Design review of the part shown in the three views and the two pictorial views. Dimensions are in mm from the part's minimum x, y and z. Give positions to 0.01 mm unless a question says otherwise; leave off trailing zeros. Loops run counter-clockwise (first coordinate to the right, second up) from the corner with the lowest first, then second, coordinate; pieces in that order, holes last. Notation, with made-up numbers: M 0,-10 L 17,-10 A22 cw 17,16 Z; hole C 46,47 d3. An arc over 180 degrees is marked long. Return JSON: item names as keys, results as strings. Group by question number.
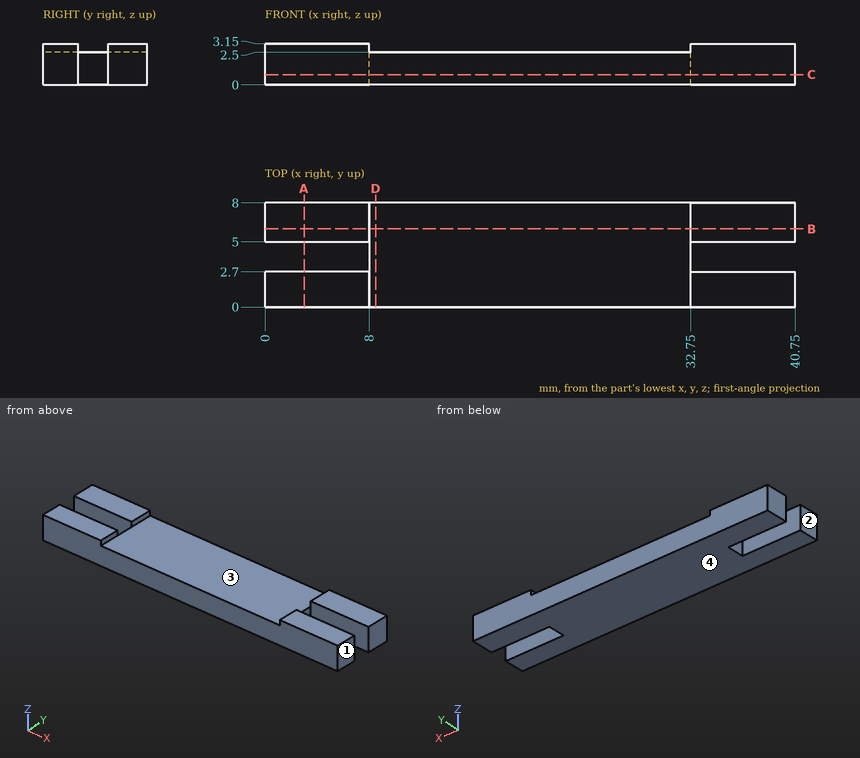
(1) For pin 1 (3 mm diameter, centred on x = 15.5, y = 6, fed in from +Z); pin 2 (1.8 mm diameter, centred on y = 3.5, z = 2, fed in from -X), all flat-tipped, find the tip position at first contact; note any pin that passes through.
(2) Add section C-C (z = 0.8). Write out the cut boundary in (x, y), and give its area (3 significant figures).
(3) For probe 1 along Y at (x, z) = (5, 0.85); probe 2 along X at (y, z) = (2.25, 2.95); probe 3 along Z at (x, y) = (19.5, 4.25), list the stretches that pass through material, from the lowest coordinate up.
(4) Add section D-D (x = 8.5). Write out the cut boundary in (y, z), and give its area (3 significant figures).
(5) Add section B-B (y = 6). Write out the cut boundary in (x, z), and give its area (3 significant figures).
(6) Mouldability with a two-part tool opening along X and no side actions: class the marked faces 1, 2, 3 and 4 as released by +X, released by -X, zero draft, split by the parting line, or undercut.
(7) Add section A-A (x = 3). Write out the cut boundary in (y, z).
Verdict:
{
 "1": {"pin 1": "stops at z = 2.5", "pin 2": "stops at x = 0"},
 "2": {"outline": "M 0,0 L 40.75,0 L 40.75,2.7 L 32.75,2.7 L 32.75,5 L 40.75,5 L 40.75,8 L 0,8 L 0,5 L 8,5 L 8,2.7 L 0,2.7 Z", "area": "289 mm²"},
 "3": {"probe 1": "y = 0 to 2.7, 5 to 8", "probe 2": "x = 0 to 8, 32.75 to 40.75", "probe 3": "z = 0 to 2.5"},
 "4": {"outline": "M 0,0 L 8,0 L 8,2.5 L 0,2.5 Z", "area": "20.0 mm²"},
 "5": {"outline": "M 0,0 L 40.75,0 L 40.75,3.15 L 32.75,3.15 L 32.75,2.5 L 8,2.5 L 8,3.15 L 0,3.15 Z", "area": "112 mm²"},
 "6": {"face 1": "released by +X", "face 2": "released by -X", "face 3": "undercut", "face 4": "zero draft"},
 "7": {"outline": "M 0,0 L 2.7,0 L 2.7,3.15 L 0,3.15 Z; M 5,0 L 8,0 L 8,3.15 L 5,3.15 Z"}
}
